Autodesk Inventor part; units mm, degrees
ref_plane "YZ Plane" through (0, 0, 0) normal (1, 0, 0) x (0, 1, 0)
ref_plane "XZ Plane" through (0, 0, 0) normal (0, 1, 0) x (-1, 0, 0)
ref_plane "XY Plane" through (0, 0, 0) normal (0, 0, 1) x (1, 0, 0)
sketch "Sketch1" plane through (0, 0, 0) normal (0, 1, 0) x (-1, 0, 0)
  line L0 (0, 0) -> (0, -415)
  line L1 (0, -415) -> (-115, -415)
  line L2 (-115, -415) -> (-115, -470)
  line L3 (-115, -470) -> (-230, -470)
  line L4 (-230, -470) -> (-345, -470) construction
  line L5 (0, 0) -> (-345, 0)
  line L6 (-345, 0) -> (-345, -355)
  line L7 (-270, -415) -> (-270, -430)
  arc A0 (-230, -470) -> (-270, -430) centre (-270.8018, -470.8018) ccw
  line L8 (-345, -355) -> (-345, -360) construction
  line L9 (-345, -360) -> (-325, -360) construction
  line L10 (-345, -360) -> (-345, -365) construction
  line L11 (-345, -365) -> (-345, -370) construction
  line L12 (-345, -370) -> (-345, -375) construction
  line L13 (-345, -375) -> (-345, -380) construction
  line L14 (-345, -365) -> (-317, -365) construction
  line L15 (-345, -370) -> (-312, -370) construction
  line L16 (-345, -375) -> (-309, -375) construction
  line L17 (-345, -380) -> (-306, -380) construction
  line L18 (-345, -380) -> (-345, -385) construction
  line L19 (-345, -385) -> (-345, -390) construction
  line L20 (-345, -390) -> (-345, -395) construction
  line L21 (-345, -395) -> (-345, -400) construction
  line L22 (-345, -400) -> (-345, -405) construction
  line L23 (-345, -405) -> (-345, -410) construction
  line L24 (-345, -385) -> (-303, -385) construction
  line L25 (-345, -390) -> (-301, -390) construction
  line L26 (-345, -395) -> (-299, -395) construction
  line L27 (-345, -400) -> (-296, -400) construction
  line L28 (-345, -405) -> (-292, -405) construction
  line L29 (-345, -410) -> (-286, -410) construction
  arc A1 (-292, -405) -> (-270, -415) centre (-268.9, -383.38) ccw
  arc A2 (-299, -395) -> (-292, -405) centre (-258.5, -374.1) ccw
  arc A3 (-299, -395) -> (-317, -365) centre (-378, -422) ccw
  arc A4 (-317, -365) -> (-345, -355) centre (-346.4167, -403.1667) ccw
  dimension "d0" = 415
  dimension "d1" = 115
  dimension "d2" = 55
  dimension "d3" = 115
  dimension "d4" = 115
  dimension "d5" = 345
  dimension "d6" = 355
  dimension "d7" = 15
  dimension "d8" = 155
  dimension "d9" = 40
  dimension "d17" = 5
  dimension "d18" = 20
  dimension "d19" = 5
  dimension "d20" = 5
  dimension "d21" = 5
  dimension "d22" = 5
  dimension "d23" = 28
  dimension "d24" = 33
  dimension "d25" = 36
  dimension "d26" = 39
  dimension "d27" = 5
  dimension "d28" = 5
  dimension "d29" = 5
  dimension "d30" = 5
  dimension "d31" = 5
  dimension "d32" = 5
  dimension "d34" = 42
  dimension "d35" = 44
  dimension "d36" = 46
  dimension "d37" = 49
  dimension "d38" = 53
  dimension "d39" = 59
  dimension "d43" = 62.5
extrude "Extrusion1" add sketch "Sketch1" along normal blind 10
sketch "Sketch2" plane through (0, 0, 0) normal (0, 0, 1) x (1, 0, 0)
  line L0 (0, 0) -> (345, 0)
  line L1 (345, 0) -> (345, 10)
  line L2 (0, 10) -> (345, 10)
  line L3 (0, 0) -> (0, 10)
extrude "Extrusion2" cut sketch "Sketch2" against normal blind 115
sketch "Sketch3" plane through (0, 10, 0) normal (0, 1, 0) x (1, 0, 0)
  line L0 (0, 115) -> (345, 115)
  line L1 (345, 115) -> (345, 355)
  arc A0 (317, 365) -> (345, 355) centre (346.4167, 403.1667) ccw
  arc A1 (299, 395) -> (317, 365) centre (378, 422) ccw
  arc A2 (299, 395) -> (292, 405) centre (258.5, 374.1) ccw
  arc A3 (292, 405) -> (270, 415) centre (268.9, 383.38) ccw
  line L2 (270, 415) -> (270, 430)
  arc A4 (230, 470) -> (270, 430) centre (270.8018, 470.8018) ccw
  line L3 (230, 470) -> (115, 470)
  line L4 (115, 470) -> (115, 415)
  line L5 (115, 415) -> (0, 415)
  line L6 (0, 415) -> (0, 115)
  point P0 (0, 0)
extrude "Extrusion3" add sketch "Sketch3" along normal blind 287
properties part number "Base Drawing"
Model file for the job. Use its own axes, mm. A direction names the side the tool comes from. Coordinates: 2 decimals unless noted, no trailing zeros. Write each loop counter-clockwise with the first axis right and the second up, starting at its lowest first coordinate (ties: lowest second). Pieces come first, ordered by that corner, then holes. Notation, with made-up numbers: (81.25, -6.75) - (127.25, -6.75) arc R22 ccw to (127.25, 6.25) - close; hole circle Ø1 at (-13.75, 69.25). An arc over 180 degrees is marked (long way). One line per item, written item: value. Start each with the question number.
1. Flat gauge pins, fed straight in: pin 1 (12 mm diameter, centred on x = 243.5, y = 90, fed in from -Z); pin 2 (12 mm diameter, centred on y = 177, z = -421.5, fed in from +X); pin 3 (2 mm diameter, centred on x = 268.5, y = 131.5, fed in from -Z); pin 4 (8 mm diameter, centred on y = 108.5, z = -303.5, fed in from -X). Where does each tip first touch, or does it go through?
2. Probe line 1 (Z direction, x = 92, y = 81.5); line 2 (Z direction, x = 320, y = 219); line 3 (X direction, y = 197.5, z = -398.5). List the from-to ranges inside material, lowest first. Write a range as from..to.
3. Slice it at A-A (y = 254). Write the cut outline in (x, z).
4. Slice it at B-B (x = 75). Write the cut outline in (y, z), plus the area to 3 significant figures.
5. Slice it at C-C (x = 238). Write the cut outline in (y, z), plus the area to 3 significant figures.
6. Tool access for faces 1 (the flat face through (175, 0, -290)), 2 (the flat face through (115, 146, -443)), 3 (the flat face through (270, 146, -422)): list every direction of +Z, -Z, +X, -X, +Y, -Y with a clear straight run to the whole face (end or side of a thin tool).
Answers below:
1. pin 1: stops at z = -447.21
1. pin 2: stops at x = 270
1. pin 3: stops at z = -430.13
1. pin 4: stops at x = 0
2. line 1: z = -415..-115
2. line 2: z = -362.87..-115
2. line 3: x = 0..296.99
3. outline: (0, -415) - (115, -415) - (115, -470) - (230, -470) arc R40.81 cw to (270, -430) - (270, -415) arc R31.64 ccw to (292, -405) arc R45.57 ccw to (299, -395) arc R83.49 cw to (317, -365) arc R48.19 cw to (345, -355) - (345, -115) - (0, -115) - close
4. outline: (0, -415) - (297, -415) - (297, -115) - (0, -115) - close
4. area: 89,100 mm^2
5. outline: (0, -446.52) - (297, -446.52) - (297, -115) - (0, -115) - close
5. area: 98,500 mm^2
6. face 1: +Z, -Z, +X, -X, -Y
6. face 2: -Z, -X, +Y, -Y
6. face 3: -Z, +X, +Y, -Y
